```python
from build123d import *

# Parameters (mm, degrees)
SKETCH1_R                = 5.5
SKETCH1_R_2              = 4.9
BOSS_EXTRUDE1_DEPTH      = 15
BOSS_EXTRUDE2_DEPTH      = 31.5
BOSS_EXTRUDE2_DEPTH_BACK = 31.5
SKETCH3_R                = 10
BOSS_EXTRUDE3_DEPTH      = 12.45
SKETCH4_R                = 10
BOSS_EXTRUDE4_DEPTH      = 12.45
CUT_EXTRUDE1_DEPTH       = 3
CUT_EXTRUDE1_DEPTH_BACK  = 3
CUT_EXTRUDE2_DEPTH       = 3
CUT_EXTRUDE2_DEPTH_BACK  = 3


with BuildPart() as part:
    # Sketch1 → Boss-Extrude1 (new body)
    with BuildSketch(Plane(origin=(0, 0, 0), x_dir=(1, 0, 0), z_dir=(0, 1, 0))):
        with BuildLine():
            Line((-23, -44.5), (23, -44.5))
            ThreePointArc((23, -44.5), (29.717514421, -41.717514421), (32.5, -35))
            Line((32.5, -35), (32.5, 35))
            ThreePointArc((32.5, 35), (29.717514421, 41.717514421), (23, 44.5))
            Line((23, 44.5), (-23, 44.5))
            ThreePointArc((-23, 44.5), (-29.717514421, 41.717514421), (-32.5, 35))
            Line((-32.5, 35), (-32.5, -35))
            ThreePointArc((-32.5, -35), (-29.717514421, -41.717514421), (-23, -44.5))
        make_face()
        with Locations((23, 35)):
            Circle(SKETCH1_R, mode=Mode.SUBTRACT)
        with Locations((23, -35)):
            Circle(SKETCH1_R, mode=Mode.SUBTRACT)
        with Locations((0, 35)):
            Circle(SKETCH1_R_2, mode=Mode.SUBTRACT)
        with Locations((0, -35)):
            Circle(SKETCH1_R_2, mode=Mode.SUBTRACT)
        with Locations((-23, 35)):
            Circle(SKETCH1_R, mode=Mode.SUBTRACT)
        with Locations((-23, -35)):
            Circle(SKETCH1_R, mode=Mode.SUBTRACT)
    extrude(amount=BOSS_EXTRUDE1_DEPTH)

    # Sketch2 → Boss-Extrude2 (add, two sides)
    with BuildSketch(Plane.XY) as boss_extrude2_sk:
        Polygon((-34.012329953, 15), (-32.7, 0), (-27.7, 0), (-27.7, 15), align=None)
    extrude(amount=BOSS_EXTRUDE2_DEPTH)
    extrude(boss_extrude2_sk.sketch, amount=-BOSS_EXTRUDE2_DEPTH_BACK)

    # Sketch3 → Boss-Extrude3 (add)
    with BuildSketch(Plane.XY.offset(25)):
        with BuildLine():
            Line((-38.215293381, 63.040091813), (-32.7, 0))
            Line((-32.7, 0), (32.5, 0))
            Line((32.5, 0), (32.5, 17.62932037))
            ThreePointArc((32.5, 17.62932037), (32.456195267, 17.989174985), (32.327339541, 18.32801182))
            Line((32.327339541, 18.32801182), (-0.302139449, 80.315885997))
            ThreePointArc((-0.302139449, 80.315885997), (-22.543503711, 90.47707817), (-37.9931465, 71.523538966))
            Line((-37.9931465, 71.523538966), (-38.215293381, 63.040091813))
        make_face()
        with Locations((-18, 71)):
            Circle(SKETCH3_R, mode=Mode.SUBTRACT)
    extrude(amount=-BOSS_EXTRUDE3_DEPTH)

    # Sketch4 → Boss-Extrude4 (add)
    with BuildSketch(Plane.XY.offset(-25)):
        with BuildLine():
            Line((-38.215293381, 63.040091813), (-32.7, 0))
            Line((-32.7, 0), (32.5, 0))
            Line((32.5, 0), (32.5, 17.62932037))
            ThreePointArc((32.5, 17.62932037), (32.456195267, 17.989174985), (32.327339541, 18.32801182))
            Line((32.327339541, 18.32801182), (-0.302139449, 80.315885997))
            ThreePointArc((-0.302139449, 80.315885997), (-22.543503711, 90.47707817), (-37.9931465, 71.523538966))
            Line((-37.9931465, 71.523538966), (-38.215293381, 63.040091813))
        make_face()
        with Locations((-18, 71)):
            Circle(SKETCH4_R, mode=Mode.SUBTRACT)
    extrude(amount=BOSS_EXTRUDE4_DEPTH)

    # Sketch5 → Cut-Extrude1 (cut, two sides)
    with BuildSketch(Plane.XY.offset(25)) as cut_extrude1_sk:
        with BuildLine():
            Line((-15.85, 57.15), (-15.85, 71))
            Line((-15.85, 71), (-20.15, 71))
            Line((-20.15, 71), (-20.15, 57.15))
            ThreePointArc((-20.15, 57.15), (-18, 55), (-15.85, 57.15))
        make_face()
    extrude(amount=CUT_EXTRUDE1_DEPTH, mode=Mode.SUBTRACT)
    extrude(cut_extrude1_sk.sketch, amount=-CUT_EXTRUDE1_DEPTH_BACK, mode=Mode.SUBTRACT)

    # Sketch6 → Cut-Extrude2 (cut, two sides)
    with BuildSketch(Plane.XY.offset(-25)) as cut_extrude2_sk:
        with BuildLine():
            Line((-15.85, 57.15), (-15.85, 71))
            Line((-15.85, 71), (-20.15, 71))
            Line((-20.15, 71), (-20.15, 57.15))
            ThreePointArc((-20.15, 57.15), (-18, 55), (-15.85, 57.15))
        make_face()
    extrude(amount=CUT_EXTRUDE2_DEPTH, mode=Mode.SUBTRACT)
    extrude(cut_extrude2_sk.sketch, amount=-CUT_EXTRUDE2_DEPTH_BACK, mode=Mode.SUBTRACT)


solid = part.part
```
Work out the finished part from the listing and answer in its coordinate system (mm). A direction names the side the tool comes from. Give positions to 0.01 mm unless a question says otherwise; leave off trailing zeros. Loops run counter-clockwise (first coordinate to the right, second up) from the corner with the lowest first, then second, coordinate; pieces in that order, holes last. Notation, with made-up numbers: (-34.75, 62) -> (6.25, 62) arc R19 cw to (6.25, 92) -> close; hole circle Ø1 at (86.25, 14). An arc over 180 degrees is marked (long way). One line per question, with ' | ' between items. Start each with the question number.
1) Section B-B, the plane y = 19.5 is taken. Determine the outline of the cut face in (x, z), then the cut area to 3 significant figures.
2) For faces 4 (the face through (0, 15, 0)), 5 (the face through (-18, 58, -22)), 6 (the face through (-32.5, 7, -33)), determine the directions among +Z, -Z, +X, -X, +Y, -Y from which every point of the face is accessible in a straight line to the end or side of a thin tool.
3) Determine the mould class of faces 1 (the face through (-32.5, 7, 33)), 2 (the face through (-17.754, 7.395, 33.348)), 3 (the face through (-22.18, 90.56, 18.86)) for opening direction X: +X half, -X half, draft (parallel to the pull), parting line (faces both ways), or undercut.
4) Section C-C, the plane y = 43 is taken. Determine the outline of the cut face in (x, z), then the cut area to 3 significant figures.
5) Each of these flat-tipped pins is pushed along its axis until it touches: pin 1 (3 mm diameter, centred on x = -15.5, z = 19.5, fed in from +Y) (3 decimals); pin 2 (2.5 mm diameter, centred on y = 59, z = -23.5, fed in from +X); pin 3 (2 mm diameter, centred on x = 1.5, y = 34, fed in from +Z); pin 4 (8 mm diameter, centred on x = 7, z = -11.5, fed in from -Y). Where does it stop, or does it pass through?
6) Section D-D, the plane z = -5.5 is taken. Determine the outline of the cut face in (x, y).
7) Section A-A, the plane y = 78 is taken. Determine the outline of the cut face in (x, z) (3 decimals), then the cut area to 3 significant figures.
8) Straight lines are drawn through the part: L1, parallel to X at y = 7, z = 35; L2, parallel to Z at x = -23, y = 3; L3, parallel to Y at x = -18, z = 22.5. For each, find the intervals that lie inside material, in ascending order.
Resolved:
1) outline: (-34.41, -25) -> (31.71, -25) -> (31.71, -12.55) -> (-34.41, -12.55) -> close; (-34.41, 12.55) -> (31.71, 12.55) -> (31.71, 25) -> (-34.41, 25) -> close | area: 1,650 mm2
2) face 4: +X, -X, +Y | face 5: -Z | face 6: -Z, -X, +Y, -Y
3) face 1: -X half | face 2: undercut | face 3: parting line
4) outline: (-36.46, -25) -> (19.34, -25) -> (19.34, -12.55) -> (-36.46, -12.55) -> close; (-36.46, 12.55) -> (19.34, 12.55) -> (19.34, 25) -> (-36.46, 25) -> close | area: 1,390 mm2
5) pin 1: y = 90.975 | pin 2: x = 11.58 | pin 3: z = 25 | pin 4: y = 0
6) outline: (-34.01, 15) -> (-32.7, 0) -> (32.5, 0) -> (32.5, 15) -> close
7) outline: (-36.735, -25) -> (-25.141, -25) -> (-25.141, -12.55) -> (-36.735, -12.55) -> close; (-36.735, 12.55) -> (-25.141, 12.55) -> (-25.141, 25) -> (-36.735, 25) -> close; (-10.859, -25) -> (0.917, -25) -> (0.917, -12.55) -> (-10.859, -12.55) -> close; (-10.859, 12.55) -> (0.917, 12.55) -> (0.917, 25) -> (-10.859, 25) -> close | area: 582 mm2
8) L1: -32.5 to -28.5, -17.5 to -4.9, 4.9 to 17.5, 28.5 to 32.5 | L2: -44.5 to -40.5, -29.5 to 29.5, 40.5 to 44.5 | L3: 0 to 55, 81 to 91
